Could you check a few things on this model? Use its own coordinates, in mm. Coordinates: 2 decimals unless noted, no trailing zeros. Write each loop counter-clockwise with the first axis right and the second up, starting at its lowest first coordinate (ties: lowest second). Pieces come first, ordered by that corner, then holes. Notation, with made-up numbers: M -40,-9 L 17,-9 A17 cw 17,3 Z; hole C 47.25,67.25 d3. An arc over 180 degrees is marked long. Write item = value, one per line.
```python
from build123d import *

# Parameters (mm, degrees)
F0_W     = 70
F0_H     = 10
F0_R     = 2
F1_DEPTH = 12
F2_W     = 70
F2_H     = 2
F3_DEPTH = 2
F4_R     = 2
F5_DEPTH = 25


with BuildPart() as f1:
    # F0 (on Top) → F1 (new body)
    with BuildSketch(Plane.XY):
        with Locations((35, -5)):
            Rectangle(F0_W, F0_H)
        with Locations((6, -5)):
            Circle(F0_R, mode=Mode.SUBTRACT)
        with Locations((64, -5)):
            Circle(F0_R, mode=Mode.SUBTRACT)
    extrude(amount=F1_DEPTH)

    # F2 (on Top) → F3 (cut)
    with BuildSketch(Plane.XY):
        with Locations((35, -1)):
            Rectangle(F2_W, F2_H)
    extrude(amount=F3_DEPTH, mode=Mode.SUBTRACT)

    # F4 (on face) → F5 (cut)
    with BuildSketch(Plane.XZ.offset(10)):
        with Locations((16, 7)):
            Circle(F4_R)
        with Locations((54, 7)):
            Circle(F4_R)
    extrude(amount=-F5_DEPTH, mode=Mode.SUBTRACT)


solid = f1.part
```
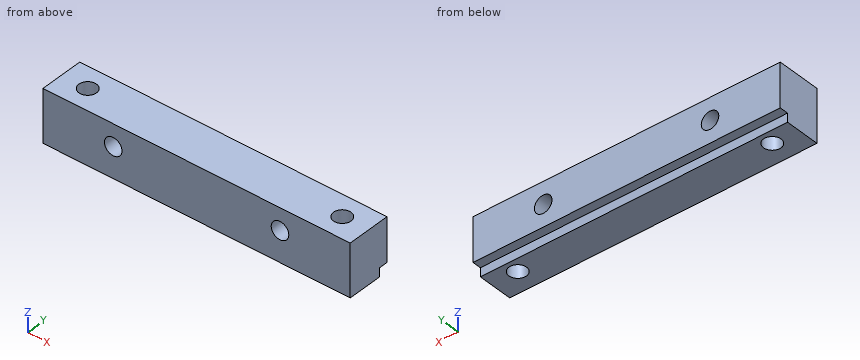
Item 1: Imagine slicing it at C-C (x = 64). Write out the boundary of the cut face in (y, z).
Numbers:
outline = M -10,0 L -7,0 L -7,12 L -10,12 Z; M -3,0 L -2,0 L -2,2 L 0,2 L 0,12 L -3,12 Z
Item 2: Imagine slicing it at A-A (z = 7). Write out the boundary of the cut face in (x, y), and give its area (3 significant figures).
Numbers:
outline = M 0,-10 L 14,-10 L 14,0 L 0,0 Z; M 18,-10 L 52,-10 L 52,0 L 18,0 Z; M 56,-10 L 70,-10 L 70,0 L 56,0 Z; hole C 6,-5 d4; hole C 64,-5 d4
area = 595 mm²
Item 3: If I drill on line 1 along Y through (x, z) = (6, 2.5); line 2 along X through (y, z) = (-4.5, 4); line 3 along Z through (x, y) = (16, -4), over which ranges is the centre line in solid material (lowest first)?
Numbers:
line_1 = -10 to -7, -3 to 0
line_2 = 0 to 4.06, 7.94 to 62.06, 65.94 to 70
line_3 = 0 to 5, 9 to 12
Item 4: Imagine slicing it at B-B (y = -6). Write out the boundary of the cut face in (x, z), and give its area (3 significant figures).
Numbers:
outline = M 0,0 L 4.27,0 L 4.27,12 L 0,12 Z; M 7.73,0 L 62.27,0 L 62.27,12 L 7.73,12 Z; M 65.73,0 L 70,0 L 70,12 L 65.73,12 Z; hole C 16,7 d4; hole C 54,7 d4
area = 732 mm²
Item 5: I'm going to push flat-ended pins straight in: P1, Ø0.6, axis at x = 37.5, z = 1.5, coming from the +Y side; P2, Ø1, axis at x = 42, y = -1, coming from the -Z side. Where does each tip first touch, or does it pass through?
Numbers:
P1 = -2
P2 = 2
Item 6: Imagine slicing it at D-D (y = -9). Write out the boundary of the cut face in (x, z).
Numbers:
outline = M 0,0 L 70,0 L 70,12 L 0,12 Z; hole C 16,7 d4; hole C 54,7 d4
